Can you work these out from the model? Positions are in its coordinate system, mm. A direction names the side the tool comes from. Give positions to 0.01 mm unless a question says otherwise; leave off trailing zeros. Write each loop counter-clockwise with the first axis right and the second up, starting at its lowest first coordinate (ties: lowest second). Pieces come first, ordered by that corner, then holes. Notation, with made-up numbers: (-30.5, 24.25) - (-8.5, 24.25) arc R6 cw to (-8.5, 35.25) - close; hole circle Ø2 at (19, 69.5). An arc over 180 degrees is marked (long way). Return JSON: item names as keys, results as strings. Group by question number.
from build123d import *

# Parameters (mm, degrees)
SKETCH_1_W          = 20
SKETCH_1_H          = 20
SKETCH_1_W_2        = 18
SKETCH_1_H_2        = 18
EXTRUDE_1_DEPTH     = 97
SKETCH_2_R          = 1.5
CUT_EXTRUDE_1_DEPTH = 166


with BuildPart() as part:
    # 草图1 → 凸台-拉伸1 (new, symmetric)
    with BuildSketch(Plane.XY):
        Rectangle(SKETCH_1_W, SKETCH_1_H)
        Rectangle(SKETCH_1_W_2, SKETCH_1_H_2, mode=Mode.SUBTRACT)
    extrude(amount=EXTRUDE_1_DEPTH, both=True)

    # 草图2 → 切除-拉伸1 (cut)
    with BuildSketch(Plane(origin=(0, 10, 0), x_dir=(1, 0, 0), z_dir=(0, 1, 0))):
        with Locations(Location((0, 87, 0), (0, 0, 270))):
            Circle(SKETCH_2_R)
        with Locations(Location((0, -87, 0), (0, 0, 270))):
            Circle(SKETCH_2_R)
        with Locations(Location((0, 0, 0), (0, 0, 270))):
            Circle(SKETCH_2_R)
        with Locations(Location((0, 15, 0), (0, 0, 270))):
            Circle(SKETCH_2_R)
        with Locations(Location((0, 30, 0), (0, 0, 270))):
            Circle(SKETCH_2_R)
        with Locations(Location((0, -30, 0), (0, 0, 270))):
            Circle(SKETCH_2_R)
        with Locations(Location((0, -15, 0), (0, 0, 270))):
            Circle(SKETCH_2_R)
    extrude(amount=-CUT_EXTRUDE_1_DEPTH, mode=Mode.SUBTRACT)


solid = part.part
1) We'd pull the mould along X, two halves only. Please class faces 3 (the face through (0.45, -9.49, -85.57)), 4 (the face through (2, 10, 1)), 5 (the face through (-10, 0, 1)): pulls with the +X half, pulls with the -X half, needs draft (parallel to the pull), parting line crosses it, or undercut.
2) I need wall thicknesses on line 1 along X through (y, z) = (0.5, -19.5); line 2 along X through (y, z) = (-9.4, 30). Which ranges of each line are inside material? Lowest first, please.
3) Imagine slicing it at B-B, the plane y = 1.5. Write out the boundary of the cut face in (x, z).
4) On a 3-axis mill with a long thin cutter (end or side, diameter ignored), from which of +Z, -Z, +X, -X, +Y, -Y can I reach the whole of each face in a straight line? I mean faces 1 (the face through (-2, -9, 1)), 2 (the face through (0.07, -9.49, -31.5)). Say none if no direction works.
5) Imagine slicing it at A-A, the plane z = 41. Write out the boundary of the cut face in (x, y).
Resolved:
{
 "1": {"face 3": "undercut", "face 4": "needs draft", "face 5": "pulls with the -X half"},
 "2": {"line 1": "-10 to -9, 9 to 10", "line 2": "-10 to -1.5, 1.5 to 10"},
 "3": {"outline": "(-10, -97) - (-9, -97) - (-9, 97) - (-10, 97) - close; (9, -97) - (10, -97) - (10, 97) - (9, 97) - close"},
 "4": {"face 1": "+Z, -Z", "face 2": "+Y, -Y"},
 "5": {"outline": "(-10, -10) - (10, -10) - (10, 10) - (-10, 10) - close; hole (-9, -9) - (9, -9) - (9, 9) - (-9, 9) - close"}
}
